Input: part model. Units: mm. Frame: model coordinates. Give positions to 0.01 mm unless a question says otherwise; leave off trailing zeros. Write each loop counter-clockwise with the first axis right and the second up, starting at its lowest first coordinate (ties: lowest second). Pieces come first, ordered by that corner, then holes. Notation, with made-up numbers: (52.25, 27.5) - (83.25, 27.5) arc R31 ccw to (83.25, 66.5) - close; hole circle Ø5 at (52, 61.5). An arc over 180 degrees is marked (long way). Use a Markdown table: item, result. Add a question column.
1. Section query B-B, the plane z = -2.55. Return loops of the section in (x, y), plus the area to 3 significant figures.
2. Section query A-A, the plane x = 203. Return loops of the section in (y, z).
3. Section query C-C, the plane y = 897.5. Return loops of the section in (x, z).
4. Material intervals for probe 1 along Y at (x, z) = (203.5, -1.7); probe 2 along X at (y, z) = (949, -1.35); probe 3 along X at (y, z) = (969, -0.6), sorted ascending.
5. Section query D-D, the plane y = 980.5. Return loops of the section in (x, z).
6. Pin query (flat end, axial travel): pin 1 (1.5 mm diameter, centred on y = 900, z = -1, fed in from +X); pin 2 (1 mm diameter, centred on x = 199, z = -2, fed in from -Y). Return the tip coordinate at first contact, or that it passes through.
```python
from build123d import *

# Parameters (mm, degrees)
ESQUISSE1_R               = 1.25
ESQUISSE1_R_2             = 1.5
ESQUISSE1_W               = 3
ESQUISSE1_H               = 5.3
T_LE_DE_BASE_PLI_E1_DEPTH = 3


# Sheet-metal steps are written as plain solids
with BuildPart() as part:
    # Esquisse1 → Tôle de base pliée1 (new body)
    with BuildSketch(Plane.XY):
        with BuildLine():
            Line((198.308869227, 952.508921018), (199.076816888, 983.793056947))
            ThreePointArc((199.076816888, 983.793056947), (202.826816888, 987.543056947), (206.576816888, 983.793056947))
            Line((206.576816888, 983.793056947), (207.344764549, 952.508921018))
            ThreePointArc((207.344764549, 952.508921018), (208.826696387, 948.522711746), (207.294357708, 944.555606441))
            Line((207.294357708, 944.555606441), (206.576816888, 868.424415079))
            ThreePointArc((206.576816888, 868.424415079), (202.826816888, 864.674415079), (199.076816888, 868.424415079))
            Line((199.076816888, 868.424415079), (198.360659982, 944.554063284))
            ThreePointArc((198.360659982, 944.554063284), (196.826944047, 948.521675361), (198.308869227, 952.508921018))
        make_face()
        with Locations((202.826816888, 983.793056947)):
            Circle(ESQUISSE1_R, mode=Mode.SUBTRACT)
        with Locations((202.826816888, 948.560738026)):
            Circle(ESQUISSE1_R_2, mode=Mode.SUBTRACT)
        with Locations((202.826816888, 868.424415079)):
            Circle(ESQUISSE1_R_2, mode=Mode.SUBTRACT)
        with Locations((202.826816888, 899.074415079)):
            Rectangle(ESQUISSE1_W, ESQUISSE1_H, mode=Mode.SUBTRACT)
    extrude(amount=-T_LE_DE_BASE_PLI_E1_DEPTH)


solid = part.part
```
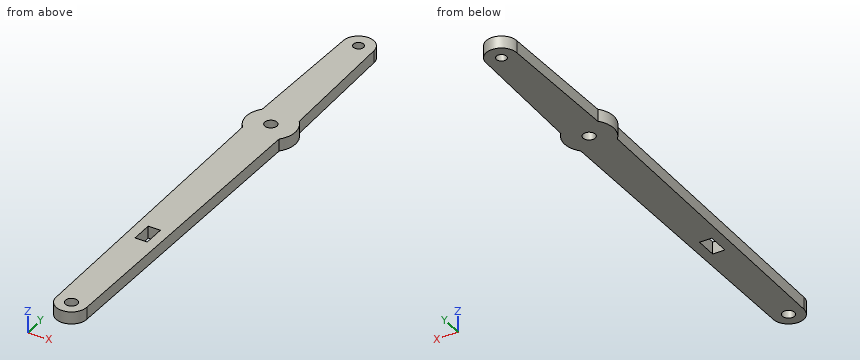
Result sheet:
| question | item | result |
|---|---|---|
| 1 | outline | (198.31, 952.51) arc R6 ccw to (198.36, 944.55) - (199.08, 868.42) arc R3.75 ccw to (206.58, 868.42) - (207.29, 944.56) arc R6 ccw to (207.34, 952.51) - (206.58, 983.79) arc R3.75 ccw to (199.08, 983.79) - close; hole circle Ø3 at (202.83, 868.42); hole (201.33, 896.42) - (204.33, 896.42) - (204.33, 901.72) - (201.33, 901.72) - close; hole circle Ø3 at (202.83, 948.56); hole circle Ø2.5 at (202.83, 983.79) |
| 1 | area | 981 mm² |
| 2 | outline | (864.68, -3) - (866.93, -3) - (866.93, 0) - (864.68, 0) - close; (869.91, -3) - (896.42, -3) - (896.42, 0) - (869.91, 0) - close; (901.72, -3) - (947.07, -3) - (947.07, 0) - (901.72, 0) - close; (950.05, -3) - (982.56, -3) - (982.56, 0) - (950.05, 0) - close; (985.03, -3) - (987.54, -3) - (987.54, 0) - (985.03, 0) - close |
| 3 | outline | (198.8, -3) - (201.33, -3) - (201.33, 0) - (198.8, 0) - close; (204.33, -3) - (206.85, -3) - (206.85, 0) - (204.33, 0) - close |
| 4 | probe 1 | y = 864.74 to 867.08, 869.76 to 896.42, 901.72 to 947.22, 949.9 to 982.74, 984.85 to 987.48 |
| 4 | probe 2 | x = 196.84 to 201.39, 204.26 to 208.81 |
| 4 | probe 3 | x = 198.71 to 206.94 |
| 5 | outline | (199, -3) - (206.66, -3) - (206.66, 0) - (199, 0) - close |
| 6 | pin 1 | stops at x = 206.88 |
| 6 | pin 2 | stops at y = 866.69 |
